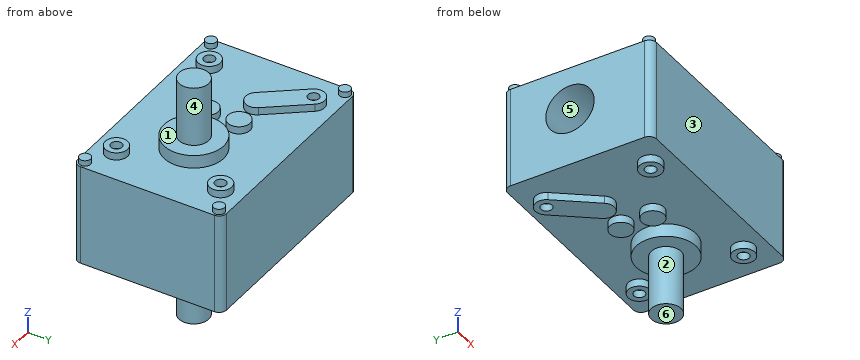
```python
from build123d import *

# Parameters (mm, degrees)
SKETCH_1_W          = 58.2
SKETCH_1_H          = 40
EXTRUDE_1_DEPTH     = 13.5
SKETCH_2_R          = 8
EXTRUDE_2_DEPTH     = 3.5
SKETCH_4_R          = 4
EXTRUDE_3_DEPTH     = 19.5
SKETCH_5_R          = 1.5
SKETCH_5_R_2        = 3
EXTRUDE_4_DEPTH     = 2
SKETCH_6_R          = 1.5
EXTRUDE_5_DEPTH     = 1.5
FILLET_1_R          = 2
SKETCH_7_R          = 6.5
CUT_EXTRUDE_1_DEPTH = 15


with BuildPart() as part:
    # 草图1 → 凸台-拉伸1 (new body)
    with BuildSketch(Plane.XY):
        Rectangle(SKETCH_1_W, SKETCH_1_H)
    extrude_1 = extrude(amount=-EXTRUDE_1_DEPTH)

    # 草图2 → 凸台-拉伸2 (add)
    with BuildSketch(Plane.XY):
        with Locations((9.1, 0)):
            Circle(SKETCH_2_R)
    extrude_2 = extrude(amount=EXTRUDE_2_DEPTH)

    # 草图4 → 凸台-拉伸3 (add)
    with BuildSketch(Plane.XY):
        with Locations((9.1, 0)):
            Circle(SKETCH_4_R)
    extrude_3 = extrude(amount=EXTRUDE_3_DEPTH)

    # 草图5 → 凸台-拉伸4 (add)
    with BuildSketch(Plane.XY):
        with BuildLine():
            Line((-9.60900018, 5.631778998), (-17.641125745, 15.853567438))
            ThreePointArc((-17.641125745, 15.853567438), (-21.853567438, 16.358874255), (-22.358874255, 12.146432562))
            Line((-22.358874255, 12.146432562), (-14.32674869, 1.924644122))
            ThreePointArc((-14.32674869, 1.924644122), (-10.114306997, 1.419337305), (-9.60900018, 5.631778998))
        make_face()
        with Locations((-20, 14)):
            Circle(SKETCH_5_R, mode=Mode.SUBTRACT)
        with Locations((20, 14)):
            Circle(SKETCH_5_R_2)
        with Locations((20, 14)):
            Circle(SKETCH_5_R, mode=Mode.SUBTRACT)
        with Locations((20, -14)):
            Circle(SKETCH_5_R_2)
        with Locations((20, -14)):
            Circle(SKETCH_5_R, mode=Mode.SUBTRACT)
        with Locations((-3.467874435, 4.285302287)):
            Circle(SKETCH_5_R_2)
        with Locations((-20, -14)):
            Circle(SKETCH_5_R_2)
        with Locations((-20, -14)):
            Circle(SKETCH_5_R, mode=Mode.SUBTRACT)
        with Locations((-3.467874435, -4.285302287)):
            Circle(SKETCH_5_R_2)
    extrude_4 = extrude(amount=EXTRUDE_4_DEPTH)

    # 镜向2: 凸台-拉伸1, 凸台-拉伸2, 凸台-拉伸3, 凸台-拉伸4 across plane
    add(extrude_1.mirror(Plane(origin=(0, 0, -13.5), x_dir=(1, 0, 0), z_dir=(0, 0, -1))))
    add(extrude_2.mirror(Plane(origin=(0, 0, -13.5), x_dir=(1, 0, 0), z_dir=(0, 0, -1))))
    add(extrude_3.mirror(Plane(origin=(0, 0, -13.5), x_dir=(1, 0, 0), z_dir=(0, 0, -1))))
    add(extrude_4.mirror(Plane(origin=(0, 0, -13.5), x_dir=(1, 0, 0), z_dir=(0, 0, -1))))

    # 草图6 → 凸台-拉伸5 (add)
    with BuildSketch(Plane.XY):
        with Locations((27.1, 18)):
            Circle(SKETCH_6_R)
        with Locations((-27.1, 18)):
            Circle(SKETCH_6_R)
        with Locations((27.1, -18)):
            Circle(SKETCH_6_R)
        with Locations((-27.1, -18)):
            Circle(SKETCH_6_R)
    extrude(amount=EXTRUDE_5_DEPTH)

    # 圆角1
    fillet_1_edges = [part.edges().sort_by_distance(p)[0] for p in [
        (29.1, -20, -13.5),
        (-29.1, -20, -13.5),
        (-29.1, 20, -13.5),
        (29.1, 20, -13.5),
    ]]
    fillet(fillet_1_edges, radius=FILLET_1_R)

    # 草图7 → 切除-拉伸1 (cut)
    with BuildSketch(Plane.ZY.offset(29.1)):
        with Locations((-11.5, 2)):
            Circle(SKETCH_7_R)
    extrude(amount=-CUT_EXTRUDE_1_DEPTH, mode=Mode.SUBTRACT)


solid = part.part
```
Source: CAD feature listing. Evaluate the final solid. Frame: model axes, mm. Face numbers are marked on the shaded views. A direction names the side the tool comes from. Give positions to 0.01 mm unless a question says otherwise; leave off trailing zeros. Order: outer loops, then holes, each group sorted by start corner. A loop starts at its lowest first (then second) coordinate and runs counter-clockwise, first axis right, second up.
(1) Section query A-A (z = -28). State how many separate pieces and enclosed holes the cut face has, plus the area to 3 significant figures.
(2) Material intervals for line 1 along Y through (x, z) = (20, 1.5); line 2 along Y through (x, z) = (-20, 0.5); line 3 along Z through (x, y) = (4.5, -8), sorted ascending.
(3) Section query D-D (x = -12). Return the cut outline in (y, z), plus the area to 3 significant figures.
(4) Pull-direction query (Y, two-part tool) for the marked faces 4, 5 and 6; classes: +Y half, -Y half, draft (parallel to the pull), parting line (faces both ways), or undercut.
(5) Contact query for flat-ended pins moving along their axis: P1, Ø2.5, axis at x = 19.5, y = 14.5, coming from the -Z side; P2, Ø1.5, axis at x = -27, y = 18, coming from the +Z side; P3, Ø2, axis at x = 16.5, z = -27.5, coming from the -Y side; P4, Ø5, axis at x = -20, y = -14, coming from the +Z side. Output: stop coordinate, or through.
(6) Access query for the marked faces 1, 2 and 3. Directions: +Z, -Z, +X, -X, +Y, -Y. A direction counts if a zero-diameter tool reaches every point of the face in a straight line with its end or side. Return the directions, or none.
(7) Section query C-C (z = -35.5). Return the cut outline in (x, y).
(8) Section query B-B (x = 9.1). Return the cut outline in (y, z), plus the area to 3 significant figures.
Outcome:
1. separate pieces: 7
1. enclosed holes: 4
1. area: 420 mm2
2. line 1: y = -17 to -15.5, -12.5 to -11, 11 to 12.5, 15.5 to 17
2. line 2: y = -17 to -15.5, -12.5 to -11, 9.14 to 12.5, 15.5 to 17
2. line 3: z = -27 to 0
3. outline: (-20, -27) - (0.78, -27) - (0.78, -29) - (8.67, -29) - (8.67, -27) - (20, -27) - (20, 0) - (8.67, 0) - (8.67, 2) - (0.78, 2) - (0.78, 0) - (-20, 0) - close
3. area: 1,110 mm2
4. face 4: parting line
4. face 5: undercut
4. face 6: draft
5. P1: stops at z = -29
5. P2: stops at z = 1.5
5. P3: stops at y = -20
5. P4: stops at z = 2
6. face 1: +Z
6. face 2: -Z
6. face 3: +Z, -Z, +X, -X, -Y
7. outline: circle Ø8 at (9.1, 0)
8. outline: (-20, -27) - (-8, -27) - (-8, -30.5) - (-4, -30.5) - (-4, -46.5) - (4, -46.5) - (4, -30.5) - (8, -30.5) - (8, -27) - (20, -27) - (20, 0) - (8, 0) - (8, 3.5) - (4, 3.5) - (4, 19.5) - (-4, 19.5) - (-4, 3.5) - (-8, 3.5) - (-8, 0) - (-20, 0) - close
8. area: 1,450 mm2
